from build123d import *

# Parameters (mm, degrees)
F0_R      = 17.85
F1_DEPTH  = 5
F4_DEPTH  = 3
F5_SIZE   = 0.635
F6_F1_R   = 5.08
F6_F2_R   = 5.08
F6_F3_R   = 5.08
F6_F4_R   = 5.08
F6_F5_R   = 5.08
F6_F6_R   = 5.08
F6_F7_R   = 5.08
F6_F8_R   = 5.08
F6_F9_R   = 5.08
F6_F10_R  = 5.08
F6_F11_R  = 5.08
F6_F12_R  = 5.08
F6_F13_R  = 5.08
F6_F14_R  = 5.08
F6_F15_R  = 5.08
F6_F16_R  = 5.08
F6_F17_R  = 5.08
F6_F18_R  = 5.08
F6_F19_R  = 5.08
F6_F20_R  = 5.08
F6_F21_R  = 5.08
F6_F22_R  = 5.08
F6_F23_R  = 5.08
F6_F24_R  = 5.08
F7_R      = 19.5
F8_DEPTH  = 1.5
F9_W      = 12.04
F9_H      = 10.6
F9_W_2    = 5.5
F9_H_2    = 3.05
F10_DEPTH = 4
F11_DEPTH = 3
F12_W     = 10
F12_H     = 1.5
F13_DEPTH = 15.1


with BuildPart() as f1:
    # F0 (on Front) → F1 (new body, symmetric)
    with BuildSketch(Plane.XZ):
        Circle(F0_R)
    extrude(amount=F1_DEPTH, both=True)

    # F3 (on offset) → F4 (join)
    with BuildSketch(Plane(origin=(0, 3, 0), x_dir=(-1, 0, 0), z_dir=(0, 1, 0))):
        Polygon((-3.2903481497, 22.4154013943), (-17.5555016387, 14.0492031865), (-21.0601798177, 8.7539476816), (-20.9370838593, -9.2984309735), (-17.1594677511, -14.4025583758), (-3.0596518503, -22.4154013943), (3.2903481497, -22.4154013943), (18.0473649217, -13.7607362086), (21.0561899697, -8.1688249226), (20.9448872454, 8.1540418144), (18.1346734923, 13.8483546493), (3.0596518503, 22.4154013943), align=None)
    extrude(amount=-F4_DEPTH)

    # F5
    f5_edges = [f1.edges().sort_by_distance(p)[0] for p in [
        (10.422925, 0, 18.232302),
        (19.307841, 0, 11.401575),
        (20.998632, 0, -0.272242),
        (19.048276, 0, -11.850495),
        (10.10956, 0, -18.40898),
        (-0.115348, 0, -22.415401),
        (-10.668857, 0, -18.088069),
        (-19.551777, 0, -10.964781),
        (-21.000539, 0, -0.007392),
        (-19.53978, 0, 11.001198),
        (-10.597163, 0, 18.131878),
        (0.115348, 0, 22.415401),
    ]]
    chamfer(f5_edges, length=F5_SIZE)

    # F6: fillet of radius 5.08 on 24 edges, made by hand

    # F6_f1
    f6_f1_edges = [f1.edges().sort_by_distance(p)[0] for p in [
        (-20.9448872454, 1.8175, 8.1540418144),
    ]]
    fillet(f6_f1_edges, radius=F6_F1_R)

    # F6_f2
    f6_f2_edges = [f1.edges().sort_by_distance(p)[0] for p in [
        (-18.1346734923, 1.8175, 13.8483546493),
    ]]
    fillet(f6_f2_edges, radius=F6_F2_R)

    # F6_f3
    f6_f3_edges = [f1.edges().sort_by_distance(p)[0] for p in [
        (-21.0561899697, 1.8175, -8.1688249226),
    ]]
    fillet(f6_f3_edges, radius=F6_F3_R)

    # F6_f4
    f6_f4_edges = [f1.edges().sort_by_distance(p)[0] for p in [
        (-20.5635101748, 0.2530156874, 8.0636856851),
    ]]
    fillet(f6_f4_edges, radius=F6_F4_R)

    # F6_f5
    f6_f5_edges = [f1.edges().sort_by_distance(p)[0] for p in [
        (-17.80801976, 0.205710524, 13.540221636),
    ]]
    fillet(f6_f5_edges, radius=F6_F5_R)

    # F6_f6
    f6_f6_edges = [f1.edges().sort_by_distance(p)[0] for p in [
        (-3.0596518503, 1.8175, 22.4154013943),
    ]]
    fillet(f6_f6_edges, radius=F6_F6_R)

    # F6_f7
    f6_f7_edges = [f1.edges().sort_by_distance(p)[0] for p in [
        (-18.0473649217, 1.8175, -13.7607362086),
    ]]
    fillet(f6_f7_edges, radius=F6_F7_R)

    # F6_f8
    f6_f8_edges = [f1.edges().sort_by_distance(p)[0] for p in [
        (-20.6589027008, 0.2383946915, -8.0701656315),
    ]]
    fillet(f6_f8_edges, radius=F6_F8_R)

    # F6_f9
    f6_f9_edges = [f1.edges().sort_by_distance(p)[0] for p in [
        (-2.9534511203, 0.2331786487, 22.013580043),
    ]]
    fillet(f6_f9_edges, radius=F6_F9_R)

    # F6_f10
    f6_f10_edges = [f1.edges().sort_by_distance(p)[0] for p in [
        (3.2903481497, 1.8175, 22.4154013943),
    ]]
    fillet(f6_f10_edges, radius=F6_F10_R)

    # F6_f11
    f6_f11_edges = [f1.edges().sort_by_distance(p)[0] for p in [
        (-3.2903481497, 1.8175, -22.4154013943),
    ]]
    fillet(f6_f11_edges, radius=F6_F11_R)

    # F6_f12
    f6_f12_edges = [f1.edges().sort_by_distance(p)[0] for p in [
        (17.5555016387, 1.8175, 14.0492031865),
    ]]
    fillet(f6_f12_edges, radius=F6_F12_R)

    # F6_f13
    f6_f13_edges = [f1.edges().sort_by_distance(p)[0] for p in [
        (3.0596518503, 1.8175, -22.4154013943),
    ]]
    fillet(f6_f13_edges, radius=F6_F13_R)

    # F6_f14
    f6_f14_edges = [f1.edges().sort_by_distance(p)[0] for p in [
        (21.0601798177, 1.8175, 8.7539476816),
    ]]
    fillet(f6_f14_edges, radius=F6_F14_R)

    # F6_f15
    f6_f15_edges = [f1.edges().sort_by_distance(p)[0] for p in [
        (17.1594677511, 1.8175, -14.4025583758),
    ]]
    fillet(f6_f15_edges, radius=F6_F15_R)

    # F6_f16
    f6_f16_edges = [f1.edges().sort_by_distance(p)[0] for p in [
        (20.9370838593, 1.8175, -9.2984309735),
    ]]
    fillet(f6_f16_edges, radius=F6_F16_R)

    # F6_f17
    f6_f17_edges = [f1.edges().sort_by_distance(p)[0] for p in [
        (-17.7394232188, 0.2231799565, -13.4639178232),
    ]]
    fillet(f6_f17_edges, radius=F6_F17_R)

    # F6_f18
    f6_f18_edges = [f1.edges().sort_by_distance(p)[0] for p in [
        (3.1799932747, 0.2286960306, 22.009097425),
    ]]
    fillet(f6_f18_edges, radius=F6_F18_R)

    # F6_f19
    f6_f19_edges = [f1.edges().sort_by_distance(p)[0] for p in [
        (17.2850276, 0.2518471741, 13.7636444987),
    ]]
    fillet(f6_f19_edges, radius=F6_F19_R)

    # F6_f20
    f6_f20_edges = [f1.edges().sort_by_distance(p)[0] for p in [
        (20.6315309968, 0.2072299177, 8.6265365553),
    ]]
    fillet(f6_f20_edges, radius=F6_F20_R)

    # F6_f21
    f6_f21_edges = [f1.edges().sort_by_distance(p)[0] for p in [
        (20.4954738766, 0.1923957856, -9.1511150124),
    ]]
    fillet(f6_f21_edges, radius=F6_F21_R)

    # F6_f22
    f6_f22_edges = [f1.edges().sort_by_distance(p)[0] for p in [
        (16.9069384559, 0.262522864, -14.1176463871),
    ]]
    fillet(f6_f22_edges, radius=F6_F22_R)

    # F6_f23
    f6_f23_edges = [f1.edges().sort_by_distance(p)[0] for p in [
        (2.9534511203, 0.2331786487, -22.013580043),
    ]]
    fillet(f6_f23_edges, radius=F6_F23_R)

    # F6_f24
    f6_f24_edges = [f1.edges().sort_by_distance(p)[0] for p in [
        (-3.1799932747, 0.2286960306, -22.009097425),
    ]]
    fillet(f6_f24_edges, radius=F6_F24_R)

    # F7 (on face) → F8 (join)
    with BuildSketch(Plane(origin=(0, 5, 0), x_dir=(-1, 0, 0), z_dir=(0, 1, 0))):
        Circle(F7_R)
    extrude(amount=F8_DEPTH)

    # F9 (on face) → F10 (join)
    with BuildSketch(Plane.XZ.offset(5)):
        Rectangle(F9_W, F9_H)
        Polygon((4.2387, -3.903), (-4.2613, -3.903), (-4.2613, 2.1469455678), (-3.0499028451, 3.877), (3.0273028451, 3.877), (4.2387, 2.1469455678), align=None, mode=Mode.SUBTRACT)
        with Locations((0, 0.9936958086)):
            Rectangle(F9_W_2, F9_H_2)
    extrude(amount=F10_DEPTH)

    # F9 (on face) → F11 (cut)
    with BuildSketch(Plane.XZ.offset(5)):
        Polygon((-4.2613, 2.1469455678), (-4.2613, -3.903), (4.2387, -3.903), (4.2387, 2.1469455678), (3.0273028451, 3.877), (-3.0499028451, 3.877), align=None)
        with Locations((0, 0.9936958086)):
            Rectangle(F9_W_2, F9_H_2, mode=Mode.SUBTRACT)
    extrude(amount=-F11_DEPTH, mode=Mode.SUBTRACT)

    # F12 (on face) → F13 (join)
    with BuildSketch(Plane(origin=(0, 6.5, 0), x_dir=(-1, 0, 0), z_dir=(0, 1, 0))):
        with BuildLine():
            Line((6.565, 3.55), (-6.565, 3.55))
            ThreePointArc((-6.565, 3.55), (-7.0140128061, 3.3640128061), (-7.2, 2.915))
            Line((-7.2, 2.915), (-7.2, -2.915))
            ThreePointArc((-7.2, -2.915), (-7.0140128061, -3.3640128061), (-6.565, -3.55))
            Line((-6.565, -3.55), (6.565, -3.55))
            ThreePointArc((6.565, -3.55), (7.0140128061, -3.3640128061), (7.2, -2.915))
            Line((7.2, -2.915), (7.2, 2.915))
            ThreePointArc((7.2, 2.915), (7.0140128061, 3.3640128061), (6.565, 3.55))
        make_face()
        with BuildLine():
            ThreePointArc((-6.95, 2.665), (-6.7640128061, 3.1140128061), (-6.315, 3.3))
            Line((-6.315, 3.3), (6.315, 3.3))
            ThreePointArc((6.315, 3.3), (6.7640128061, 3.1140128061), (6.95, 2.665))
            Line((6.95, 2.665), (6.95, -2.665))
            ThreePointArc((6.95, -2.665), (6.7640128061, -3.1140128061), (6.315, -3.3))
            Line((6.315, -3.3), (-6.315, -3.3))
            ThreePointArc((-6.315, -3.3), (-6.7640128061, -3.1140128061), (-6.95, -2.665))
            Line((-6.95, -2.665), (-6.95, 2.665))
        make_face(mode=Mode.SUBTRACT)
        with Locations((0, 0.7)):
            Rectangle(F12_W, F12_H)
    extrude(amount=F13_DEPTH)


solid = f1.part
Could you check a few things on this model? Use its own coordinates, in mm. A direction names the side the tool comes from. Give positions to 0.01 mm unless a question says otherwise; leave off trailing zeros. Loops run counter-clockwise (first coordinate to the right, second up) from the corner with the lowest first, then second, coordinate; pieces in that order, holes last. Notation, with made-up numbers: (24, 7.5) -> (59, 7.5) arc R18 ccw to (59, 25.5) -> close; hole circle Ø7 at (85, -26.75). An arc over 180 degrees is marked (long way). Answer as CSV lines item,"result". Start each with the question number.
(1) I need wall thicknesses on probe 1 along Z at (x, y) = (-2.5, 17.5); probe 2 along Y at (x, z) = (15.5, 11); probe 3 along Y at (x, z) = (-5, 10.5). Which ranges of each line are inside material? Lowest first, please.
(2) I'm going to push flat-ended pins straight in: pin 1 Ø3.5 at (y, z) = (-5.5, 0.5) entering from +X; pin 2 Ø6.5 at (y, z) = (-7, -2) entering from -X; pin 3 Ø12 at (x, y) = (0.5, 17.5) entering from +Z. Where does each tip first touch, or does it pass through?
(3) If we section it at D-D on x = -11: Write out the boundary of the cut face in (y, z) (3 decimals), then the cut area to 3 significant figures.
(4) If we section it at A-A on y = 16: Write out the boundary of the cut face in (x, z) (3 decimals), then the cut area to 3 significant figures.
(5) We'd pull the mould along X, two halves only. Please class faces 1 (the cylindrical face through (17.096, 1.782, -14.309)), 2 (the cylindrical face through (-17.92, 1.77, -13.61)), 3 (the flat face through (-9, 5, -16)), 4 (the flat face through (0, 14, 1.45)): released by +X, released by -X, zero draft, split by the parting line, or undercut.
(6) If we section it at C-C on y = 4: Write out the boundary of the cut face in (x, z).
(7) Which directions (+Z, -Z, +X, -X, +Y, -Y) give clear straight access to the entire face, cutting with the end or side of a thin tool? Please do faces 5 (the flat face through (0, 14, -3.55)), 6 (the flat face through (6.95, 14, 0)), 7 (the flat face through (-3.664, -5.451, 3)).
(8) If we section it at B-B on x = 13.5: Write out the boundary of the cut face in (y, z) (3 decimals).
Computed:
1,probe 1,"z = -3.55 to -3.3, -0.05 to 1.45, 3.3 to 3.55"
1,probe 2,"y = 0 to 3, 5 to 6.5"
1,probe 3,"y = -5 to 6.5"
2,pin 1,"stops at x = 17.85"
2,pin 2,"stops at x = -17.85"
2,pin 3,"stops at z = 3.55"
3,outline,"(-5, -14.058) -> (0, -14.058) -> (0, -17.158) -> (0.635, -17.894) -> (3, -17.894) -> (3, -14.058) -> (5, -14.058) -> (5, -16.101) -> (6.5, -16.101) -> (6.5, 16.101) -> (5, 16.101) -> (5, 14.058) -> (3, 14.058) -> (3, 17.903) -> (0.635, 17.903) -> (0, 17.173) -> (0, 14.058) -> (-5, 14.058) -> close"
3,area,"352 mm2"
4,outline,"(-7.2, -2.915) arc R0.635 ccw to (-6.565, -3.55) -> (6.565, -3.55) arc R0.635 ccw to (7.2, -2.915) -> (7.2, 2.915) arc R0.635 ccw to (6.565, 3.55) -> (-6.565, 3.55) arc R0.635 ccw to (-7.2, 2.915) -> close; (-5, -0.05) -> (5, -0.05) -> (5, 1.45) -> (-5, 1.45) -> close; hole (-6.95, -2.665) arc R0.635 ccw to (-6.315, -3.3) -> (6.315, -3.3) arc R0.635 ccw to (6.95, -2.665) -> (6.95, 2.665) arc R0.635 ccw to (6.315, 3.3) -> (-6.315, 3.3) arc R0.635 ccw to (-6.95, 2.665) -> close"
4,area,"25.5 mm2"
5,face 1,"released by +X"
5,face 2,"released by -X"
5,face 3,"zero draft"
5,face 4,"undercut"
6,outline,"circle Ø35.7 at (0, 0)"
7,face 5,"-Z, +X, -X, +Y"
7,face 6,"+Y"
7,face 7,"-Y"
8,outline,"(-5, -11.678) -> (0, -11.678) -> (0, -15.752) -> (0.635, -16.482) -> (3, -16.482) -> (3, -11.678) -> (5, -11.678) -> (5, -14.071) -> (6.5, -14.071) -> (6.5, 14.071) -> (5, 14.071) -> (5, 11.678) -> (3, 11.678) -> (3, 16.428) -> (0.635, 16.428) -> (0, 15.692) -> (0, 11.678) -> (-5, 11.678) -> close"
